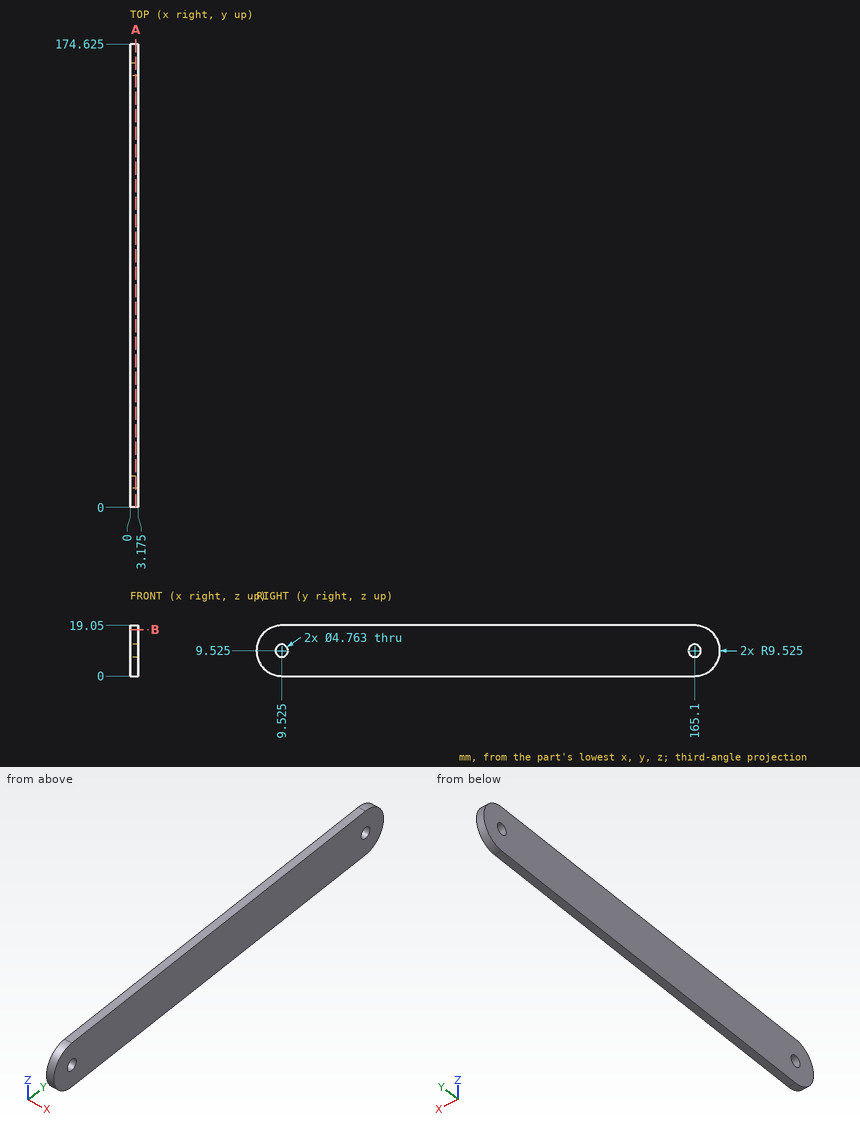
Check sheet for the drawn part. Datum: minimum x, y, z corner. Units: mm. Round coordinates to 2 decimals unless told otherwise and drop trailing zeros. Loops run counter-clockwise (first coordinate to the right, second up) from the corner with the lowest first, then second, coordinate; pieces in that order, holes last. Notation, with made-up numbers: (2, 84.25) - (49, 84.25) arc R20 ccw to (49, 123.25) - close; hole circle Ø3 at (52, 1). An arc over 180 degrees is marked (long way). Use one line per item in the form item = value.
1. Scan lines: probe 1 along Y at (x, z) = (0.2, 9.5) (1 decimal); probe 2 along Z at (x, y) = (1.3, 165.1); probe 3 along Y at (x, z) = (0.4, 7) (1 decimal). Record each from-to range of solid material in increasing order.
A:
probe_1 = 0 to 7.1, 11.9 to 162.7, 167.5 to 174.6
probe_2 = 0 to 7.14, 11.91 to 19.05
probe_3 = 0.3 to 174.3
2. Gauge pin test, flat ends, axial feed: pin 1 Ø3 at (y, z) = (9.525, 9.525) entering from -X; pin 2 Ø1.5 at (x, z) = (2.5, 8) entering from -Y; pin 3 Ø1.5 at (x, z) = (1.5, 16) entering from -Y. Record the tip position at first contact, or that the pin passes through.
A:
pin_1 = through
pin_2 = 0.03
pin_3 = 1.91
3. Section check A-A on x = 2.2. Give the number of separate pieces and of enclosed holes in the cut face, and give its area (3 significant figures).
A:
separate_pieces = 1
enclosed_holes = 2
area = 3,210 mm²
4. Section check B-B on z = 17.5. Record the cut outline in (x, y) (1 decimal).
A:
outline = (0, 4.3) - (3.2, 4.3) - (3.2, 170.3) - (0, 170.3) - close
